Autodesk Inventor part; units mm, degrees
ref_plane "YZ Plane" through (0, 0, 0) normal (1, 0, 0) x (0, 1, 0)
ref_plane "XZ Plane" through (0, 0, 0) normal (0, 1, 0) x (-1, 0, 0)
ref_plane "XY Plane" through (0, 0, 0) normal (0, 0, 1) x (1, 0, 0)
sketch "Block1" plane through (0, 0, 0) normal (0, 0, 1) x (1, 0, 0)
  circle A0 centre (74.029, 24.2723) radius 1
  line L0 (49.279, 30.4723) -> (71.779, 30.4723)
  line L1 (71.779, 30.4723) -> (71.779, 18.0723)
  line L2 (71.779, 18.0723) -> (49.279, 18.0723)
  line L3 (49.279, 18.0723) -> (49.279, 30.4723)
  line L4 (49.279, 30.4723) -> (44.779, 30.4723)
  line L5 (44.779, 30.4723) -> (44.779, 18.0723)
  line L6 (44.779, 18.0723) -> (49.279, 18.0723)
  line L7 (49.279, 18.0723) -> (49.279, 30.4723)
  line L8 (71.779, 30.4723) -> (76.279, 30.4723)
  line L9 (76.279, 30.4723) -> (76.279, 18.0723)
  line L10 (76.279, 18.0723) -> (71.779, 18.0723)
  line L11 (71.779, 18.0723) -> (71.779, 30.4723)
  line L12 (44.779, 24.2723) -> (76.279, 24.2723) construction
  line L13 (47.029, 30.4723) -> (47.029, 18.0723) construction
  circle A1 centre (47.029, 24.2723) radius 1
  line L14 (74.029, 30.4723) -> (74.029, 18.0723) construction
  point P0 (60.979, 24.0984)
  dimension "d7" = 22.5
  dimension "d8" = 12.4
  dimension "d9" = 4.5
  dimension "d10" = 4.5
  dimension "d11" = 2
  dimension "d12" = 2
sketch "Sketch1" plane through (0, 0, 0) normal (0, 0, 1) x (1, 0, 0)
  line L0 (-54.534, 30.732) -> (-16.034, 30.732)
  line L1 (-16.034, 30.732) -> (-16.034, 23.732)
  line L2 (-16.034, 23.732) -> (-54.534, 23.732)
  line L3 (-54.534, 23.732) -> (-54.534, 30.732)
  line L4 (-92.7646, -8.503) -> (-89.7646, -8.503)
  line L5 (-89.7646, -8.503) -> (-89.7646, -11.753)
  line L6 (-89.7646, -11.753) -> (-92.7646, -11.753)
  line L7 (-92.7646, -11.753) -> (-92.7646, -8.503)
  line L8 (-92.7646, -21.6527) -> (-89.7646, -21.6527)
  line L9 (-89.7646, -21.6527) -> (-89.7646, -21.7527)
  line L10 (-89.7646, -21.7527) -> (-92.7646, -21.7527)
  line L11 (-92.7646, -21.7527) -> (-92.7646, -21.6527)
  line L12 (-48.784, 23.732) -> (-21.784, 23.732)
  line L13 (-21.784, 23.732) -> (-21.784, -13.768)
  line L14 (-21.784, -13.768) -> (-48.784, -13.768)
  line L15 (-48.784, -13.768) -> (-48.784, 23.732)
  line L16 (-35.284, 30.732) -> (-35.284, 23.732) construction
  line L17 (-35.284, -13.768) -> (-35.284, 23.732) construction
  circle A0 centre (-35.284, 18.482) radius 1
  line L18 (-41.484, -6.268) -> (-41.484, 16.232)
  line L19 (-41.484, 16.232) -> (-29.084, 16.232)
  line L20 (-29.084, 16.232) -> (-29.084, -6.268)
  line L21 (-29.084, -6.268) -> (-41.484, -6.268)
  line L22 (-41.484, -6.268) -> (-41.484, -10.768)
  line L23 (-41.484, -10.768) -> (-29.084, -10.768)
  line L24 (-29.084, -10.768) -> (-29.084, -6.268)
  line L25 (-29.084, -6.268) -> (-41.484, -6.268)
  line L26 (-41.484, 16.232) -> (-41.484, 20.732)
  line L27 (-41.484, 20.732) -> (-29.084, 20.732)
  line L28 (-29.084, 20.732) -> (-29.084, 16.232)
  line L29 (-29.084, 16.232) -> (-41.484, 16.232)
  line L30 (-35.284, -10.768) -> (-35.284, 20.732) construction
  line L31 (-41.484, -8.518) -> (-29.084, -8.518) construction
  circle A1 centre (-35.284, -8.518) radius 1
  line L32 (-41.484, 18.482) -> (-29.084, 18.482) construction
  point P0 (0, 0)
  dimension "d0" = 3
  dimension "mat" = 3.25
  dimension "d2" = 3
  dimension "d3" = 0.1
  dimension "d4" = 38.5
  dimension "d6" = 7
  dimension "d15" = 3
  dimension "d17" = 27
  dimension "d19" = 3
  dimension "d20" = 37.5
extrude "Extrusion1" add sketch "Sketch1" along normal blind 3.25 contours L0 L1 L2 L3 | L2 L13 L14 L15 | L21 L24 L23 L22 | L26 L27 L28 L19
equation "\"d21\" = mat"
properties part number "arm-servo"
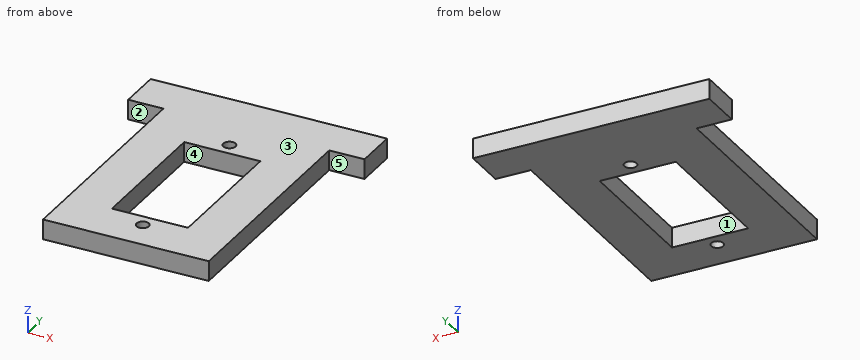
Read the model definition and answer for the solid it produces. Units are mm, in the model's axes. Face numbers are marked on the shaded views. A direction names the side the tool comes from. Round coordinates to 2 decimals unless told otherwise and drop trailing zeros. Write each loop counter-clockwise with the first axis right and the second up, starting at its lowest first coordinate (ties: lowest second). Pieces come first, ordered by that corner, then holes. Notation, with made-up numbers: M -2.75,45 L 24.25,45 A20 cw 24.25,72 Z; hole C -38,5.5 d6. An arc over 180 degrees is marked long. One line per item, written item: value.
Q1. For a pull along X with two mould halves and no side action, classify the marked faces 4 and 5 as +X half, -X half, draft (parallel to the pull), parting line (faces both ways), or undercut.
Data:
face 4: undercut
face 5: draft
Q2. Find section C-C on z = 1.65. Write down the section's boundary in (x, y), plus the area to 3 significant figures.
Data:
outline: M -54.53,23.73 L -48.78,23.73 L -48.78,-13.77 L -21.78,-13.77 L -21.78,23.73 L -16.03,23.73 L -16.03,30.73 L -54.53,30.73 Z; hole M -41.48,-6.27 L -29.08,-6.27 L -29.08,16.23 L -41.48,16.23 Z; hole C -35.28,-8.52 d2; hole C -35.28,18.48 d2
area: 997 mm2
Q3. Find section B-B on y = 3. Write down the section's boundary in (x, z).
Data:
outline: M -48.78,0 L -41.48,0 L -41.48,3.25 L -48.78,3.25 Z; M -29.08,0 L -21.78,0 L -21.78,3.25 L -29.08,3.25 Z
Q4. Find section A-A on x = -30.5. Write down the section's boundary in (y, z), plus the area to 3 significant figures.
Data:
outline: M -13.77,0 L -6.27,0 L -6.27,3.25 L -13.77,3.25 Z; M 16.23,0 L 30.73,0 L 30.73,3.25 L 16.23,3.25 Z
area: 71.5 mm2
Q5. Flat-ended cylindrical pins translate along their axes: pin 1 Ø1 at (y, z) = (0, 2) entering from +X; pin 2 Ø1 at (y, z) = (14, 0.5) entering from -X. Find the tip coordinate at first contact, or state that the pin passes through.
Data:
pin 1: x = -21.78
pin 2: x = -48.78
Q6. Straight lines are drawn through the part: line 1 (X direction, y = 14.5, z = 0.8); line 2 (Y direction, x = -35, z = 1.6); line 3 (Y direction, x = -34.5, z = 0.6). For each, find the intervals that lie inside material, in ascending order. Write a range as [from, to].
Data:
line 1: [-48.78, -41.48], [-29.08, -21.78]
line 2: [-13.77, -9.48], [-7.56, -6.27], [16.23, 17.52], [19.44, 30.73]
line 3: [-13.77, -9.14], [-7.9, -6.27], [16.23, 17.86], [19.1, 30.73]
Q7. Which of the six approach directions +Z, -Z, +X, -X, +Y, -Y give full straight-line access (tool end or side, diameter ignored) to the marked faces 1, 2 and 3?
Data:
face 1: +Z, -Z
face 2: +Z, -Z, -X, -Y
face 3: +Z, +X, -X, +Y, -Y
